Check sheet for the modelled part. Datum: model origin and axes. Units: mm. A direction names the side the tool comes from. Give positions to 0.01 mm unless a question says otherwise; leave off trailing zeros. Order: outer loops, then holes, each group sorted by start corner. A loop starts at its lowest first (then second) coordinate and runs counter-clockwise, first axis right, second up.
Item 1: Sectioned sample at B-B on z = 8.5. Record the boundary of the cut face in (x, y).
Item 2: Gauge pin test, flat ends, axial feed: P1, Ø1.5, axis at x = 5.5, z = 11.5, coming from the -Y side; P2, Ø2.5, axis at y = 1, z = 9.5, coming from the -X side; P3, Ø3.5, axis at y = 1, z = 10, coming from the +X side. Record the tip position at first contact, or that the pin passes through.
Item 3: Sectioned sample at C-C on z = 11. Record the boundary of the cut face in (x, y), and give its area (3 significant figures).
Item 4: Access from +Z, -Z, +X, -X, +Y, -Y to the whole of each face (thin tool, end or side, straight path). Record for faces 5 (the flat face through (-5.716, 0, 10)), 6 (the cylindrical face through (3.3, 0.1, 6.9)), 7 (the cylindrical face through (9, 0, 9)).
Item 5: Release check for a two-part mould opening along Y. For faces 1 (the cylindrical face through (-4.57, 7.167, 12.592)), 2 (the flat face through (2.82, 4.97, 9.73)), 3 (the flat face through (9, 0, 12)), 4 (the flat face through (-2.82, -4.97, 9.73)) record: released by +Y, released by -Y, zero draft, split by the parting line, or undercut.
Item 6: Material ranges on line 1 along Y through (x, z) = (0, 7); line 2 along Y through (x, z) = (0, 12.4); line 3 along Z through (x, y) = (-3, -5), recorded low to high.
Item 7: Sectioned sample at A-A on y = 0. Record the boundary of the cut face in (x, z), and give its area (3 significant figures).
Item 8: Sectioned sample at D-D on z = 12.75. Record the boundary of the cut face in (x, y).
from build123d import *

# Parameters (mm, degrees)
SKETCH002_R             = 9
SKETCH002_R_2           = 3.3
EXTRUDE001_DEPTH        = 1
SKETCH003_R             = 8.5
SKETCH003_R_2           = 7.5
EXTRUDE003_DEPTH        = 1.2
SKETCH001_R             = 9
EXTRUDE002_DEPTH        = 4.6
BODY003_PLACEMENT_ANGLE = 180


with BuildPart() as extrude001:
    # Sketch002 → Extrude001 (new body)
    with BuildSketch(Plane.XY):
        Circle(SKETCH002_R)
        Circle(SKETCH002_R_2, mode=Mode.SUBTRACT)
    extrude(amount=EXTRUDE001_DEPTH)


with BuildPart() as extrude001_1:
    # Extrude001 placement: moved
    add(extrude001.part.moved(Location((0, 0, 4.6))))


with BuildPart() as extrude003:
    # Sketch003 → Extrude003 (new body)
    with BuildSketch(Plane.XY):
        Circle(SKETCH003_R)
        Circle(SKETCH003_R_2, mode=Mode.SUBTRACT)
    extrude(amount=-EXTRUDE003_DEPTH)


with BuildPart() as revolve_body:
    # Sketch007 → Revolve (revolve)
    with BuildSketch(Plane.XZ):
        Polygon((-9, 1.4), (-9, 0), (-10.4, 0), align=None)
    revolve(axis=Axis((0, 0, 0), (0, 0, 1)))


with BuildPart() as body003:
    # Sketch001 → Extrude002 (new body)
    with BuildSketch(Plane.XY):
        Circle(SKETCH001_R)
        Polygon((5.715768, 3.3), (0, 6.6), (-5.715768, 3.3), (-5.715768, -3.3), (0, -6.6), (5.715768, -3.3), align=None, mode=Mode.SUBTRACT)
    extrude(amount=EXTRUDE002_DEPTH)

    # Fusion: union Extrude001, Extrude003, Revolve body
    add(extrude001_1.part)
    add(extrude003.part)
    add(revolve_body.part)


with BuildPart() as body003_1:
    # Body003 placement: moved
    add(body003.part.moved(Location((0, 0, 12))).rotate(Axis((0, 0, 12), (0, 1, 0)), BODY003_PLACEMENT_ANGLE))


solid = body003_1.part
Report:
1. outline: circle Ø18 at (0, 0); hole (-5.72, -3.3) - (0, -6.6) - (5.72, -3.3) - (5.72, 3.3) - (0, 6.6) - (-5.72, 3.3) - close
2. P1: stops at y = -9.15
2. P2: stops at x = -9.1
2. P3: stops at x = 10.11
3. outline: circle Ø18.8 at (0, 0); hole (-5.72, -3.3) - (0, -6.6) - (5.72, -3.3) - (5.72, 3.3) - (0, 6.6) - (-5.72, 3.3) - close
3. area: 164 mm2
4. face 5: +Z
4. face 6: +Z, -Z
4. face 7: -Z
5. face 1: split by the parting line
5. face 2: undercut
5. face 3: zero draft
5. face 4: undercut
6. line 1: y = -9 to -3.3, 3.3 to 9
6. line 2: y = -8.5 to -7.5, 7.5 to 8.5
6. line 3: z = 6.4 to 12
7. outline: (-10.4, 12) - (-9, 10.6) - (-9, 6.4) - (-3.3, 6.4) - (-3.3, 7.4) - (-5.72, 7.4) - (-5.72, 12) - (-7.5, 12) - (-7.5, 13.2) - (-8.5, 13.2) - (-8.5, 12) - close; (3.3, 6.4) - (9, 6.4) - (9, 10.6) - (10.4, 12) - (8.5, 12) - (8.5, 13.2) - (7.5, 13.2) - (7.5, 12) - (5.72, 12) - (5.72, 7.4) - (3.3, 7.4) - close
7. area: 46.0 mm2
8. outline: circle Ø17 at (0, 0); hole circle Ø15 at (0, 0)
